```python
from build123d import *

# Parameters (mm, degrees)
BOSS_EXTRU_1_DEPTH       = 2
ESQUISSE2_R              = 1.6
ENL_V_MAT_EXTRU_1_DEPTH  = 155.04220201
CONG_1_R                 = 10
ESQUISSE5_W              = 20
ESQUISSE5_H              = 37
ENL_V_MAT_EXTRU_4_DEPTH  = 10
ESQUISSE6_W              = 4
ESQUISSE6_H              = 40
BOSS_EXTRU_3_DEPTH       = 14.5
ESQUISSE10_W             = 12.3
ESQUISSE10_H             = 4.5
ENL_V_MAT_EXTRU_5_DEPTH  = 12.1
ESQUISSE9_W              = 13
ESQUISSE9_H              = 38
ENL_V_MAT_EXTRU_6_DEPTH  = 3
ESQUISSE11_W             = 2.2
ESQUISSE11_H             = 13
ENL_V_MAT_EXTRU_7_DEPTH  = 3
ESQUISSE14_R             = 6.45
BOSS_EXTRU_4_DEPTH       = 20
ESQUISSE15_R             = 5.45
ENL_V_MAT_EXTRU_8_DEPTH  = 156.592416268
ESQUISSE17_W             = 30
ESQUISSE17_H             = 100
ENL_V_MAT_EXTRU_10_DEPTH = 156.32224567
ESQUISSE18_W             = 2.5
ESQUISSE18_H             = 4.5
BOSS_EXTRU_5_DEPTH       = 32
ESQUISSE19_R             = 1.55
ENL_V_MAT_EXTRU_11_DEPTH = 177.567975579


with BuildPart() as part:
    # Esquisse1 → Boss.-Extru.1 (new body)
    with BuildSketch(Plane.XY):
        Polygon((100, -90), (125, -90), (125, 90), (100, 90), (100, 65), (48, 65), (48, 90), (-48, 90), (-48, 65), (-100, 65), (-100, 90), (-125, 90), (-125, -90), (-100, -90), (-100, -65), (-48, -65), (-48, -90), (48, -90), (48, -65), (100, -65), align=None)
    extrude(amount=-BOSS_EXTRU_1_DEPTH)

    # Esquisse2 → Enlèv. mat.-Extru.1 (cut, through all)
    with BuildSketch(Plane(origin=(0, 0, -2), x_dir=(-1, 0, 0), z_dir=(0, 0, -1))):
        with Locations((-118.55, 78.76)):
            Circle(ESQUISSE2_R)
        with Locations(Location((118.55, 78.76, 0), (0, 0, 180))):
            Circle(ESQUISSE2_R)
        with Locations((118.55, -78.76)):
            Circle(ESQUISSE2_R)
        with Locations(Location((-118.55, -78.76, 0), (0, 0, 180))):
            Circle(ESQUISSE2_R)
    extrude(amount=-ENL_V_MAT_EXTRU_1_DEPTH, mode=Mode.SUBTRACT)

    # Congé1
    cong_1_edges = [part.edges().sort_by_distance(p)[0] for p in [
        (-100, 90, -1),
        (-48, 90, -1),
        (-48, 65, -1),
        (-100, 65, -1),
        (100, 65, -1),
        (48, 65, -1),
        (48, 90, -1),
        (100, 90, -1),
        (48, -90, -1),
        (48, -65, -1),
        (100, -65, -1),
        (100, -90, -1),
        (-100, -65, -1),
        (-48, -65, -1),
        (-48, -90, -1),
        (-100, -90, -1),
        (125, 90, -1),
        (125, -90, -1),
        (-125, -90, -1),
        (-125, 90, -1),
    ]]
    fillet(cong_1_edges, radius=CONG_1_R)

    # Esquisse5 → Enlèv. mat.-Extru.4 (cut)
    with BuildSketch(Plane(origin=(0, 0, -2), x_dir=(-1, 0, 0), z_dir=(0, 0, -1))):
        with Locations((-90, 0)):
            Rectangle(ESQUISSE5_W, ESQUISSE5_H)
    extrude(amount=-ENL_V_MAT_EXTRU_4_DEPTH, mode=Mode.SUBTRACT)

    # Esquisse6 → Boss.-Extru.3 (add)
    with BuildSketch(Plane.XY):
        with Locations((120, 44)):
            Rectangle(ESQUISSE6_W, ESQUISSE6_H)
    extrude(amount=BOSS_EXTRU_3_DEPTH)

    # Esquisse10 → Enlèv. mat.-Extru.5 (cut)
    with BuildSketch(Plane(origin=(122, 0, 0), x_dir=(0, 0, -1), z_dir=(1, 0, 0))):
        with Locations((-7.25, 60.15)):
            Rectangle(ESQUISSE10_W, ESQUISSE10_H)
    extrude(amount=-ENL_V_MAT_EXTRU_5_DEPTH, mode=Mode.SUBTRACT)

    # Esquisse9 → Enlèv. mat.-Extru.6 (cut)
    with BuildSketch(Plane(origin=(122, 0, 0), x_dir=(0, 0, -1), z_dir=(1, 0, 0))):
        with Locations((-6.5, 44)):
            Rectangle(ESQUISSE9_W, ESQUISSE9_H)
    extrude(amount=-ENL_V_MAT_EXTRU_6_DEPTH, mode=Mode.SUBTRACT)

    # Esquisse11 → Enlèv. mat.-Extru.7 (cut)
    with BuildSketch(Plane(origin=(0, 25, 0), x_dir=(1, 0, 0), z_dir=(0, 1, 0))):
        with Locations((120, -6.5)):
            Rectangle(ESQUISSE11_W, ESQUISSE11_H)
    extrude(amount=-ENL_V_MAT_EXTRU_7_DEPTH, mode=Mode.SUBTRACT)

    # Esquisse14 → Boss.-Extru.4 (add)
    with BuildSketch(Plane.XY):
        with Locations(Location((116.644469063, 0, 0), (0, 0, 180))):
            Circle(ESQUISSE14_R)
    extrude(amount=BOSS_EXTRU_4_DEPTH)

    # Esquisse15 → Enlèv. mat.-Extru.8 (cut, through all)
    with BuildSketch(Plane.XY.offset(20)):
        with Locations((116.644469063, 0)):
            Circle(ESQUISSE15_R)
    extrude(amount=-ENL_V_MAT_EXTRU_8_DEPTH, mode=Mode.SUBTRACT)

    # Esquisse17 → Enlèv. mat.-Extru.10 (cut, through all)
    with BuildSketch(Plane.XY):
        with Locations((-74, 0)):
            Rectangle(ESQUISSE17_W, ESQUISSE17_H)
    extrude(amount=-ENL_V_MAT_EXTRU_10_DEPTH, mode=Mode.SUBTRACT)

    # Esquisse18 → Boss.-Extru.5 (add)
    with BuildSketch(Plane.XY):
        with Locations((-22.25, 0)):
            Rectangle(ESQUISSE18_W, ESQUISSE18_H)
        with Locations((22.25, 0)):
            Rectangle(ESQUISSE18_W, ESQUISSE18_H)
    extrude(amount=BOSS_EXTRU_5_DEPTH)

    # Esquisse19 → Enlèv. mat.-Extru.11 (cut, through all)
    with BuildSketch(Plane(origin=(23.5, 0, 0), x_dir=(0, 0, -1), z_dir=(1, 0, 0))):
        with Locations((-28.5, 0)):
            Circle(ESQUISSE19_R)
    extrude(amount=-ENL_V_MAT_EXTRU_11_DEPTH, mode=Mode.SUBTRACT)


solid = part.part
```
Geometry: final body of the model. Coordinates: model frame, mm. A direction names the side the tool comes from. Give positions to 0.01 mm unless a question says otherwise; leave off trailing zeros. Loops run counter-clockwise (first coordinate to the right, second up) from the corner with the lowest first, then second, coordinate; pieces in that order, holes last. Notation, with made-up numbers: (-34, 73.25) -> (-28, 73.25) arc R27 ccw to (-28, 103.25) -> close; hole circle Ø5 at (16.25, -20.75). An arc over 180 degrees is marked (long way). Use one line per item in the form item = value.
Item 1: Section query B-B on z = 4.5. Output: boundary loops of the cut face in (x, y), and give its area (3 significant figures).
A:
outline = (-23.5, -2.25) -> (-21, -2.25) -> (-21, 2.25) -> (-23.5, 2.25) -> close; (21, -2.25) -> (23.5, -2.25) -> (23.5, 2.25) -> (21, 2.25) -> close; circle Ø12.9 at (116.64, 0); (118, 24) -> (118.9, 24) -> (118.9, 25) -> (119, 25) -> (119, 57.9) -> (118, 57.9) -> close; (118, 62.4) -> (119, 62.4) -> (119, 63) -> (122, 63) -> (122, 64) -> (118, 64) -> close; (121.1, 24) -> (122, 24) -> (122, 25) -> (121.1, 25) -> close; hole circle Ø10.9 at (116.64, 0)
area = 99.2 mm^2
Item 2: Section query C-C on y = 70.5. Output: boundary loops of the cut face in (x, z), and give its area (3 significant figures).
A:
outline = (-125, -2) -> (-98.93, -2) -> (-98.93, 0) -> (-125, 0) -> close; (-49.07, -2) -> (49.07, -2) -> (49.07, 0) -> (-49.07, 0) -> close; (98.93, -2) -> (125, -2) -> (125, 0) -> (98.93, 0) -> close
area = 301 mm^2
Item 3: Access query for faces 1 (the face through (51.01, -67.85, -1.01)), 2 (the face through (122, 44, 14)), 3 (the face through (-96.99, 67.85, -1.01)). Directions: +Z, -Z, +X, -X, +Y, -Y. A direction counts if a zero-diameter tool reaches every point of the face in a straight line with its end or side. Return the directions, or none.
A:
face_1 = +Z, -Z, -Y
face_2 = +Z, +X, +Y
face_3 = +Z, -Z, +Y
Item 4: Section query D-D on x = -29.5. Output: boundary loops of the cut face in (y, z).
A:
outline = (-90, -2) -> (90, -2) -> (90, 0) -> (-90, 0) -> close
Item 5: Section query A-A on y = -69. Output: boundary loops of the cut face in (x, z).
A:
outline = (-125, -2) -> (-98, -2) -> (-98, 0) -> (-125, 0) -> close; (-50, -2) -> (50, -2) -> (50, 0) -> (-50, 0) -> close; (98, -2) -> (125, -2) -> (125, 0) -> (98, 0) -> close
Item 6: Line query: probe 1 along X at (y, z) = (-78.76, -0.6); probe 2 along Y at (x, z) = (-22.3, 28.5); probe 3 along Y at (x, z) = (-118.55, -0.75). Output: solid intervals per line, ascending.
A:
probe_1 = -125 to -120.15, -116.95 to -100, -48 to 48, 100 to 116.95, 120.15 to 125
probe_2 = -2.25 to -1.55, 1.55 to 2.25
probe_3 = -89.35 to -80.36, -77.16 to 77.16, 80.36 to 89.35
Item 7: Pin query (flat end, axial travel): P1, Ø10, axis at x = -32, z = 17.5, coming from the -Y side; P2, Ø2, axis at x = 22, z = 22, coming from the +Y side; P3, Ø8, axis at x = -86.5, y = 31.5, coming from the -Z side; P4, Ø0.8, axis at x = 118.5, y = 60, coming from the +Z side. Return the tip coordinate at first contact, or that it passes through.
A:
P1 = through
P2 = 2.25
P3 = -2
P4 = 14.5
Item 8: Draft query along X for faces 4 (the face through (-2, 1, -2)), 5 (the face through (121.99, -87.15, -1.01)), 6 (the face through (45.15, 86.99, -1.01)). Return one class per face: pulls with the +X half, pulls with the -X half, needs draft (parallel to the pull), parting line crosses it, or undercut.
A:
face_4 = needs draft
face_5 = pulls with the +X half
face_6 = undercut
